Design review of the part built by this model. Coordinates are the model's own, in mm. A direction names the side the tool comes from. Coordinates: 2 decimals unless noted, no trailing zeros. Order: outer loops, then holes, each group sorted by start corner. A loop starts at its lowest first (then second) coordinate and runs counter-clockwise, first axis right, second up. Notation, with made-up numbers: M 25,-23.5 L 63,-23.5 A5 ccw 63,-17.5 Z; hole C -1.5,74 d3. An arc over 180 degrees is marked long. Answer in a Markdown table with one row per item.
Autodesk Inventor part; units mm, degrees
ref_plane "YZ Plane" through (0, 0, 0) normal (1, 0, 0) x (0, 1, 0)
ref_plane "XZ Plane" through (0, 0, 0) normal (0, 1, 0) x (-1, 0, 0)
ref_plane "XY Plane" through (0, 0, 0) normal (0, 0, 1) x (1, 0, 0)
sketch "Sketch1" plane through (0, 0, 0) normal (0, 0, 1) x (1, 0, 0)
  circle A0 centre (0, 0) radius 13.1
  line L0 (0, 0) -> (-8.5876, 9.8926)
  line L1 (-8.5876, 9.8926) -> (-10.5542, 12.1581)
  circle A1 centre (0, 0) radius 16.1
  point P0 (0, 0)
  dimension "d0" = 3
extrude "Extrusion1" add sketch "Sketch1" against normal blind 28.2
sketch "Sketch2" plane through (0, 0, 0) normal (0, 0, 1) x (1, 0, 0)
  circle A0 centre (0, 0) radius 13.1
  point P0 (0, 0)
extrude "Extrusion2" add sketch "Sketch2" against normal blind 2.85
sketch "Sketch4" plane through (0, 0, -28.2) normal (0, 0, -1) x (-1, 0, 0)
  circle A0 centre (0, 0) radius 16.1
  circle A1 centre (0, 0) radius 13.1
  circle A2 centre (0, 0) radius 12.5
  point P0 (0, 0)
extrude "Extrusion3" add sketch "Sketch4" along normal blind 2.6 contours A0 | A1
properties part number "opona"
(1) Insertion check: pin 1 Ø3 at (y, z) = (-1, -5.5) entering from +X; pin 2 Ø10 at (y, z) = (-11, -25.5) entering from +X; pin 3 Ø8 at (x, z) = (12.5, -6) entering from -Y; pin 4 Ø8 at (x, y) = (-4, -1) entering from -Z. Each pin has a flat end and moves straight along its axis. Give the tip position at first contact, or say it passes through.
Return value:
| item | result |
|---|---|
| pin 1 | stops at x = 16.1 |
| pin 2 | stops at x = 14.94 |
| pin 3 | stops at y = -13.67 |
| pin 4 | stops at z = -2.85 |
(2) For faces 1 (the cylindrical face through (-1.705, 12.989, -15.348)), 2 (the flat face through (0, 0, 0)), 3 (the cylindrical face through (-11.923, -3.755, -29.482)), list the 3-axis set-ups (+Z, -Z, +X, -X, +Y, -Y) from which the entire face can be reached by the end or side of a thin tool; tool diameter is ignored.
Return value:
| item | result |
|---|---|
| face 1 | none |
| face 2 | +Z, +X, -X, +Y, -Y |
| face 3 | -Z |
(3) Add section A-A, the plane y = 0. Give the boundary of the cut face in (x, z).
Return value:
| item | result |
|---|---|
| outline | M -16.1,-30.8 L -12.5,-30.8 L -12.5,-28.2 L -13.1,-28.2 L -13.1,-2.85 L 13.1,-2.85 L 13.1,-28.2 L 12.5,-28.2 L 12.5,-30.8 L 16.1,-30.8 L 16.1,0 L -16.1,0 Z |
(4) Add section C-C, the plane z = -17.5. Give the boundary of the cut face in (x, y).
Return value:
| item | result |
|---|---|
| outline | C 0,0 d32.2; hole C 0,0 d26.2 |
(5) For line 1 along Z through (x, y) = (5.5, 11.5); line 2 along Y through (x, z) = (0, -29.4); line 3 along Y through (x, z) = (0, -28), list the stretches that pass through material, from the lowest coordinate up. Write a range as from..to.
Return value:
| item | result |
|---|---|
| line 1 | z = -30.8..-28.2, -2.85..0 |
| line 2 | y = -16.1..-12.5, 12.5..16.1 |
| line 3 | y = -16.1..-13.1, 13.1..16.1 |
(6) Add section D-D, the plane y = 14. Give the boundary of the cut face in (x, z).
Return value:
| item | result |
|---|---|
| outline | M -7.95,-30.8 L 7.95,-30.8 L 7.95,0 L -7.95,0 Z |
(7) Draft analysis for pull direction Y (two halves, no side actions). For faces 4 (the flat face through (0, 0, -2.85)), 5 (the flat face through (-5, -12, -30.8)), state which applies: pulls with the +Y half, pulls with the -Y half, needs draft (parallel to the pull), parting line crosses it, or undercut.
Return value:
| item | result |
|---|---|
| face 4 | undercut |
| face 5 | needs draft |
